Read the model definition and answer for the solid it produces. Units are mm, in the model's axes. A direction names the side the tool comes from. Give positions to 0.01 mm unless a question says otherwise; leave off trailing zeros. Order: outer loops, then holes, each group sorted by start corner. A loop starts at its lowest first (then second) coordinate and runs counter-clockwise, first axis right, second up. Notation, with made-up numbers: (-22, 78) - (-14, 78) arc R16 ccw to (-14, 105) - close; hole circle Ø2 at (57, 43). An arc over 180 degrees is marked (long way). Write item = value, one per line.
```python
from build123d import *

# Parameters (mm, degrees)
F0_W     = 50.8
F0_H     = 19.05
F1_DEPTH = 1123.95
F2_W     = 122.435573
F2_H     = 50.8
F2_W_2   = 108.831619
F2_W_3   = 93.867282
F2_W_4   = 145.562325
F2_W_5   = 343.160421
F2_H_2   = 127
F2_W_6   = 155.851283
F3_DEPTH = 25.4
F4_R     = 0.79375
F5_DEPTH = 25.4
F6_R     = 4.7625
F7_DEPTH = 25.4


with BuildPart() as f1:
    # F0 (on Top) → F1 (new body)
    with BuildSketch(Plane.XY):
        Rectangle(F0_W, F0_H)
    extrude(amount=F1_DEPTH)

    # F2 (on Front) → F3 (cut)
    with BuildSketch(Plane.XZ):
        with Locations((22.446524, 25.4)):
            Rectangle(F2_W, F2_H)
        with Locations((-4.761385, 342.9)):
            Rectangle(F2_W_2, F2_H)
        with Locations((2.720783, 755.65)):
            Rectangle(F2_W_3, F2_H)
        with Locations((-1.360391, 444.5)):
            Rectangle(F2_W_4, F2_H)
        with Locations((-38.781822, 1060.45)):
            Rectangle(F2_W_5, F2_H_2)
        with Locations((-12.806606, 254)):
            Rectangle(F2_W_6, F2_H)
    extrude(amount=F3_DEPTH, mode=Mode.SUBTRACT)

    # F4 (on Front) → F5 (cut)
    with BuildSketch(Plane.XZ):
        with Locations((9.525, 101.6)):
            Circle(F4_R)
        with Locations((9.525, 155.575)):
            Circle(F4_R)
        with Locations((9.525, 625.475)):
            Circle(F4_R)
        with Locations((9.525, 679.45)):
            Circle(F4_R)
        with Locations((-9.525, 625.475)):
            Circle(F4_R)
        with Locations((-9.525, 679.45)):
            Circle(F4_R)
        with Locations((-9.525, 101.6)):
            Circle(F4_R)
        with Locations((-9.525, 155.575)):
            Circle(F4_R)
    extrude(amount=-F5_DEPTH, mode=Mode.SUBTRACT)

    # F6 (on Front) → F7 (cut)
    with BuildSketch(Plane.XZ):
        with Locations((15.875, 254)):
            Circle(F6_R)
        with Locations((-15.875, 254)):
            Circle(F6_R)
        with Locations((-15.875, 482.6)):
            Circle(F6_R)
    extrude(amount=F7_DEPTH, mode=Mode.SUBTRACT)


solid = f1.part
```
1. For faces 3 (the face through (0, 0, 254)), 4 (the face through (0, 0, 1061)), 5 (the face through (0, 0, 26)), determine the directions among +Z, -Z, +X, -X, +Y, -Y from which every point of the face is accessible in a straight line to the end or side of a thin tool.
Recorded:
face_3 = +X, -X, -Y
face_4 = +Z, +X, -X, -Y
face_5 = -Z, +X, -X, -Y
2. Determine the mould class of faces 1 (the face through (0, -9.525, 598)), 2 (the face through (0, 0, 445)) for opening direction Z: +Z half, -Z half, draft (parallel to the pull), parting line (faces both ways), or undercut.
Recorded:
face_1 = draft
face_2 = undercut
3. Section A-A (z = 1025) is taken. Determine the outline of the cut face in (x, y) (3 decimals).
Recorded:
outline = (-25.4, 0) - (25.4, 0) - (25.4, 9.525) - (-25.4, 9.525) - close
4. Straight lines are drawn through the part: L1, parallel to X at y = 3.75, z = 101.6; L2, parallel to Z at x = -3.5, y = -0.5; L3, parallel to Y at x = -11, z = 237.5 (3 decimals). For each, find the intervals that lie inside material, in ascending order. Write a range as [from, to].
Recorded:
L1 = [-25.4, -10.32], [-8.73, 8.73], [10.32, 25.4]
L2 = [50.8, 228.6], [279.4, 317.5], [368.3, 419.1], [469.9, 730.25], [781.05, 996.95]
L3 = [0, 9.525]
5. Flat-ended cylindrical pins translate along their axes: pin 1 (3 mm diameter, centred on x = 8, y = -7, fed in from -Z); pin 2 (1.3 mm diameter, centred on x = -9.525, z = 679.45, fed in from +Y); pin 3 (1.5 mm diameter, centred on x = 4, z = 754, fed in from -Y); pin 4 (5 mm diameter, centred on y = -3.5, z = 424, fed in from -X). Find the tip coordinate at first contact, or state that the pin passes through.
Recorded:
pin_1 = 50.8
pin_2 = 0
pin_3 = 0
pin_4 = through
